from build123d import *

# Parameters (mm, degrees)
F0_R            = 25
F0_R_2          = 22
F1_DEPTH        = 15
F3_DEPTH        = 15
F3_COPIES_COUNT = 4
F5_R            = 38.565863123
F5_R_2          = 23
F6_DEPTH        = 2.5
F7_R            = 30.9780307995
F7_R_2          = 23
F8_DEPTH        = 4


# Not quite as in the source:
# - a pattern or mirror of a feature is missing from the dataset's text; its kind, count and spacing are read off the source's solid


with BuildPart() as f1:
    # F0 (on Top) → F1 (new body)
    with BuildSketch(Plane.XY):
        Circle(F0_R)
        Circle(F0_R_2, mode=Mode.SUBTRACT)
    extrude(amount=F1_DEPTH)

    # F2 (on Top) → F3 (cut, through all)
    with BuildSketch(Plane.XY):
        with BuildLine():
            Line((13.1922580361, 18.8404970186), (14.3394109088, 20.4788011072))
            ThreePointArc((14.3394109088, 20.4788011072), (6.4704761276, 24.1481456572), (-2.1788935687, 24.9048674523))
            Line((-2.1788935687, 24.9048674523), (-2.0045820832, 22.9124780561))
            ThreePointArc((-2.0045820832, 22.9124780561), (5.9528380374, 22.2162940046), (13.1922580361, 18.8404970186))
        make_face()
    f3 = extrude(amount=F3_DEPTH, mode=Mode.SUBTRACT)

    # F3_copies: F3 ×4 about axis
    f3_copies_axis = Axis((0, 0, 0), (0, 0, 1))
    for i in range(1, F3_COPIES_COUNT):
        add(f3.rotate(f3_copies_axis, i * 360 / F3_COPIES_COUNT), mode=Mode.SUBTRACT)

    # F5 (on offset) → F6 (cut, symmetric)
    with BuildSketch(Plane.XY.offset(7.5)):
        Circle(F5_R)
        Circle(F5_R_2, mode=Mode.SUBTRACT)
    extrude(amount=F6_DEPTH, both=True, mode=Mode.SUBTRACT)

    # F7 (on face) → F8 (cut)
    with BuildSketch(Plane.XY.offset(5)):
        Circle(F7_R)
        Circle(F7_R_2, mode=Mode.SUBTRACT)
    extrude(amount=-F8_DEPTH, mode=Mode.SUBTRACT)


solid = f1.part
Can you work these out from the model? Positions are in its coordinate system, mm. A direction names the side the tool comes from. Give positions to 0.01 mm unless a question says otherwise; leave off trailing zeros. Order: outer loops, then holes, each group sorted by start corner. A loop starts at its lowest first (then second) coordinate and runs counter-clockwise, first axis right, second up. Notation, with made-up numbers: M 73,8 L 85,8 A17 cw 85,35 Z; hole C 31.5,67.5 d6. An arc over 180 degrees is marked long. One line per item, written item: value.
Item 1: Please list where these lines run through material, in increasing order: line 1 (X direction, y = 15.5, z = 12.75); line 2 (X direction, y = 6.5, z = 3.25); line 3 (Y direction, x = 19.5, z = 13).
Verdict:
line 1: -19.62 to -15.61, 15.61 to 19.62
line 2: -22.06 to -21.02, 21.02 to 22.06
line 3: -15.64 to -13.65, -12.2 to -10.19, 10.19 to 15.64
Item 2: If we mould it in two halves opening along Y, with no side actions, what happens to faces 1 (the face through (-19.65, 13.76, 12.46)), 2 (the face through (13.76, 19.65, 0.49)), 3 (the face through (20, 12, 10))? For each: pulls with the +Y half, pulls with the -Y half, needs draft (parallel to the pull), parting line crosses it, or undercut.
Verdict:
face 1: undercut
face 2: pulls with the +Y half
face 3: needs draft
Item 3: If we section it at A-A on x = 0: Write out the boundary of the cut face in (y, z).
Verdict:
outline: M -23,0 L -22,0 L -22,15 L -23,15 Z; M 22,0 L 23,0 L 23,15 L 22,15 Z
Item 4: If we section it at D-D on z = 11.5: Write out the boundary of the cut face in (x, y), and give its area (3 significant figures).
Verdict:
outline: M -24.9,-2.18 A25 ccw -14.34,-20.48 L -13.19,-18.84 A23 ccw 2,-22.91 L 2.18,-24.9 A25 ccw 20.48,-14.34 L 18.84,-13.19 A23 ccw 22.91,2 L 24.9,2.18 A25 ccw 14.34,20.48 L 13.19,18.84 A23 ccw -2,22.91 L -2.18,24.9 A25 ccw -20.48,14.34 L -18.84,13.19 A23 ccw -22.91,-2 Z; hole C 0,0 d44
area: 309 mm2
Item 5: For faces 4 (the face through (-13.76, -19.65, 12.46)), 5 (the face through (13.76, 19.65, 12.46)), 6 (the face through (20, 12, 1)), 7 (the face through (12, -20, 10)), 8 (the face through (-20.4, -11.2, 1)), which set-ups out of +Z, -Z, +X, -X, +Y, -Y let a thin tool reach every point of the face, with its end or its side?
Verdict:
face 4: +Z, -Z, -Y
face 5: +Z, -Z, +Y
face 6: +X, +Y
face 7: +X, -Y
face 8: -X, -Y
Item 6: If we section it at B-B on z = 7.25: Write out the boundary of the cut face in (x, y).
Verdict:
outline: C 0,0 d46; hole C 0,0 d44
Item 7: For pin 1 (1.5 mm diameter, centred on x = -10, z = 9, fed in from +Y); pin 2 (1 mm diameter, centred on x = 9.5, z = 10, fed in from -Y); pin 3 (3.5 mm diameter, centred on x = 10.5, y = -16, fed in from +Z); pin 4 (5 mm diameter, centred on x = -11, z = 9, fed in from +Y), each with a flat end and sliding along its axis, tell me the tip position at first contact or that it passes through.
Verdict:
pin 1: y = 21.06
pin 2: y = -23.32
pin 3: through
pin 4: y = 23.43
